Check sheet for the drawn part. Datum: minimum x, y, z corner. Units: mm. Round coordinates to 2 decimals unless told otherwise and drop trailing zeros. Order: outer loops, then holes, each group sorted by start corner. A loop starts at its lowest first (then second) coordinate and runs counter-clockwise, first axis right, second up. Notation, with made-up numbers: M 42.5,58.5 L 89.5,58.5 A33 cw 89.5,87.5 Z; hole C -37.5,-17.5 d10. An arc over 180 degrees is marked long. Use one line per item in the form item = value. Start each with the question number.
Item 1: Cross-section at A-A on x = 1880. Enter the section's corners in (y, z).
Item 2: Thickness scan on probe 1 along X at (y, z) = (880, 26); probe 2 along Y at (x, z) = (1880, 13); probe 3 along X at (y, z) = (143, 10). Record the ranges inside material, lowest first. Write a range as [from, to].
Item 3: Cross-section at B-B on y = 880. Enter the section's corners in (x, z), then the cut area to 3 significant figures.
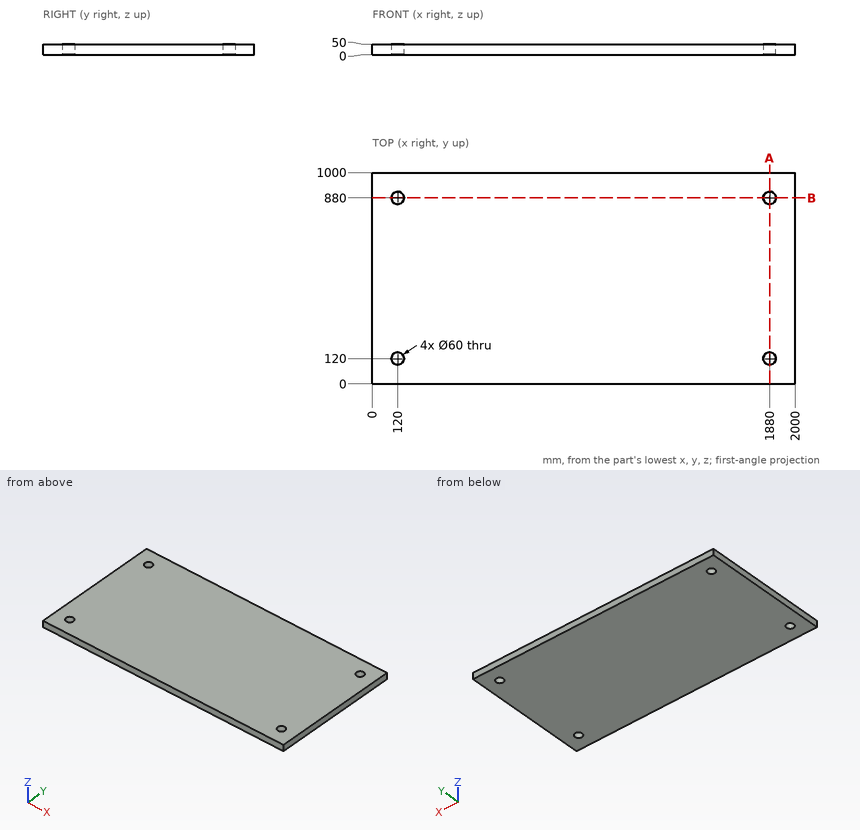
Output values:
q1.outline = M 0,0 L 90,0 L 90,50 L 0,50 Z; M 150,0 L 850,0 L 850,50 L 150,50 Z; M 910,0 L 1000,0 L 1000,50 L 910,50 Z
q2.probe_1 = [0, 90], [150, 1850], [1910, 2000]
q2.probe_2 = [0, 90], [150, 850], [910, 1000]
q2.probe_3 = [0, 100.74], [139.26, 1860.74], [1899.26, 2000]
q3.outline = M 0,0 L 90,0 L 90,50 L 0,50 Z; M 150,0 L 1850,0 L 1850,50 L 150,50 Z; M 1910,0 L 2000,0 L 2000,50 L 1910,50 Z
q3.area = 94,000 mm2
